Verification items for this drawing (mm, ordinates from the low corner). A direction names the side the tool comes from. Give positions to 0.01 mm unless a question says otherwise; leave off trailing zeros. Loops run counter-clockwise (first coordinate to the right, second up) from the corner with the lowest first, then second, coordinate; pieces in that order, holes last. Notation, with made-up numbers: (-6.5, 36) -> (15.5, 36) arc R11 ccw to (15.5, 42) -> close; hole circle Ø10 at (-17, 27.25). An arc over 180 degrees is marked (long way). Use one line per item in the form item = value. Start each with the question number.
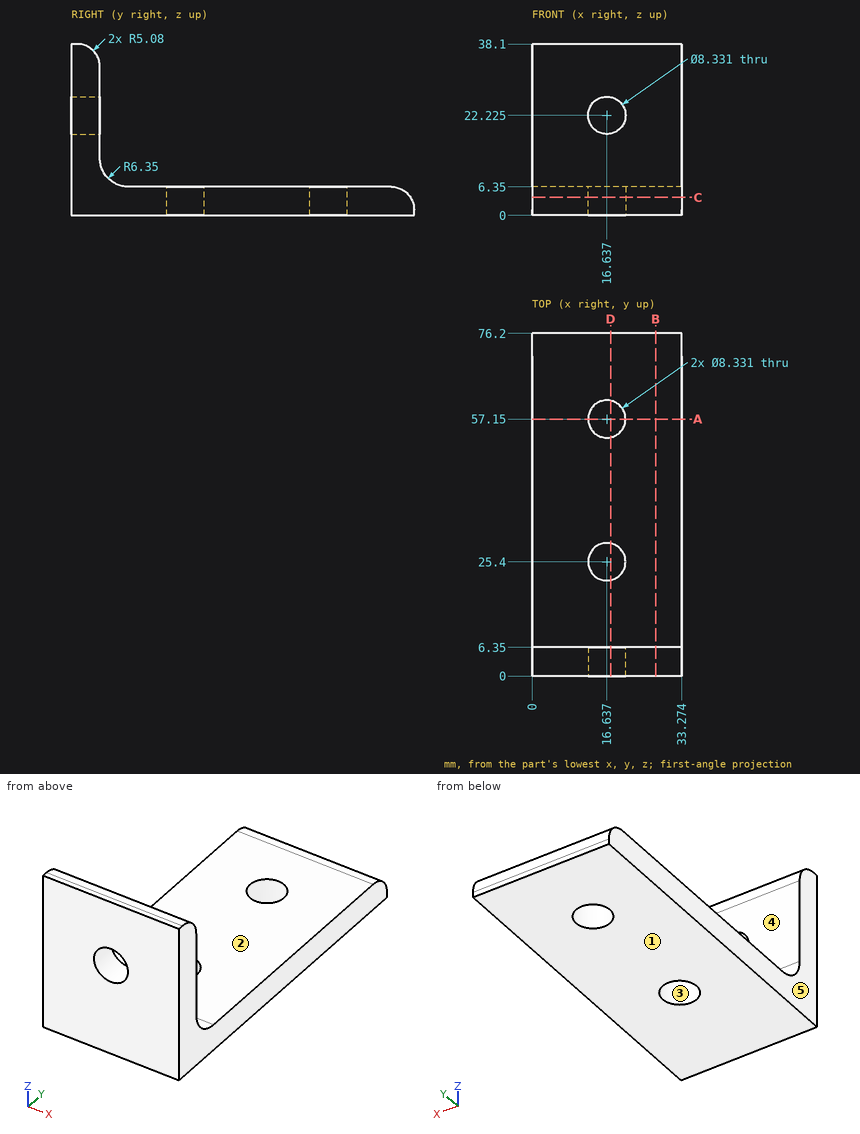
Item 1: Sectioned sample at C-C, the plane z = 4. Enter the section's corners in (x, y), and give its area (3 significant figures).
Item 2: Draft check along Y on the marked faces 3, 4 and 5. Enter one of: +Y half, -Y half, draft (parallel to the pull), parting line (faces both ways), or undercut.
Item 3: Sectioned sample at B-B, the plane x = 27.5. Enter the section's corners in (y, z).
Item 4: Tool access check on the marked faces 1 and 2. Record the directions out of +Z, -Z, +X, -X, +Y, -Y that give a thin tool (end or side, any length) a straight path to the whole face; none if there is none.
Item 5: Sectioned sample at D-D, the plane x = 17.5. State how many separate pieces and enclosed holes the cut face has, and give its area (3 significant figures).
Item 6: Material ranges on line 1 (Y direction, x = 31.5, z = 22), recorded low to high.
Item 7: Sectioned sample at A-A, the plane y = 57.15. Enter the section's corners in (x, z).
Item 8: Gauge pin test, flat ends, axial feed: pin 1 Ø10 at (x, z) = (11, 22.5) entering from +Y; pin 2 Ø3 at (x, y) = (14.5, 44) entering from +Z. Record the tip position at first contact, or that the pin passes through.
Outcome:
q1.outline = (0, 0) -> (33.27, 0) -> (33.27, 75.4) -> (0, 75.4) -> close; hole circle Ø8.33 at (16.64, 25.4); hole circle Ø8.33 at (16.64, 57.15)
q1.area = 2,400 mm^2
q2.face_3 = undercut
q2.face_4 = +Y half
q2.face_5 = draft
q3.outline = (0, 0) -> (76.2, 0) -> (76.2, 1.27) arc R5.08 ccw to (71.12, 6.35) -> (12.7, 6.35) arc R6.35 cw to (6.35, 12.7) -> (6.35, 33.02) arc R5.08 ccw to (1.27, 38.1) -> (0, 38.1) -> close
q4.face_1 = -Z, +X, -X, +Y, -Y
q4.face_2 = +Z, +X, -X, +Y
q5.separate_pieces = 4
q5.enclosed_holes = 0
q5.area = 528 mm^2
q6.line_1 = 0 to 6.35
q7.outline = (0, 0) -> (12.47, 0) -> (12.47, 6.35) -> (0, 6.35) -> close; (20.8, 0) -> (33.27, 0) -> (33.27, 6.35) -> (20.8, 6.35) -> close
q8.pin_1 = 6.35
q8.pin_2 = 6.35
